from build123d import *

# Parameters (mm, degrees)
F1_DEPTH = 7


with BuildPart() as f1:
    # F0 (on Top) → F1 (new body)
    with BuildSketch(Plane.XY):
        with BuildLine():
            Line((41.277483, 14.2875), (0, 14.2875))
            ThreePointArc((0, 14.2875), (-7.9375, 6.35), (0, -1.5875))
            Line((0, -1.5875), (41.277483, -1.5875))
            ThreePointArc((41.277483, -1.5875), (49.214983, 6.35), (41.277483, 14.2875))
        make_face()
        with BuildLine():
            Line((41.277483, 0), (0, 0))
            ThreePointArc((0, 0), (-6.35, 6.35), (0, 12.7))
            Line((0, 12.7), (41.277483, 12.7))
            ThreePointArc((41.277483, 12.7), (47.627483, 6.35), (41.277483, 0))
        make_face(mode=Mode.SUBTRACT)
    extrude(amount=F1_DEPTH)


solid = f1.part
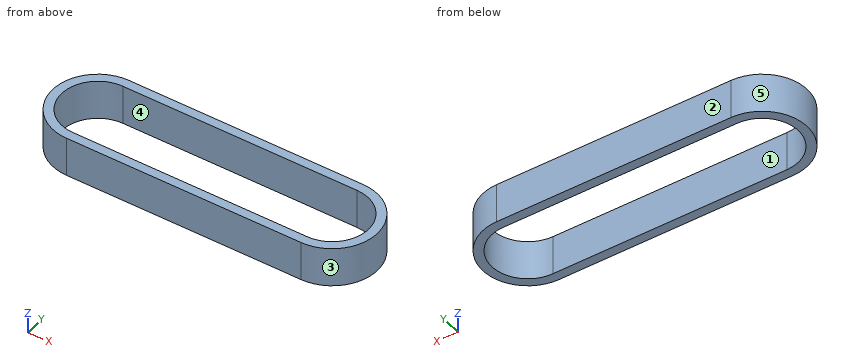
Could you check a few things on this model? Use its own coordinates, in mm. Face numbers are marked on the shaded views. A direction names the side the tool comes from. Round coordinates to 2 decimals unless told otherwise and drop trailing zeros. Loops run counter-clockwise (first coordinate to the right, second up) from the corner with the lowest first, then second, coordinate; pieces in that order, holes last. Notation, with made-up numbers: (-10, 1) - (2, 1) arc R15 ccw to (2, 30) - close; hole circle Ø9 at (-12, 9). An arc over 180 degrees is marked (long way). Write item = value, one per line.
1) Imagine slicing it at A-A (y = 6.35). Please give me the cut outline in (x, z), and give its area (3 significant figures).
Computed:
outline = (-7.94, 0) - (-6.35, 0) - (-6.35, 7) - (-7.94, 7) - close; (47.63, 0) - (49.21, 0) - (49.21, 7) - (47.63, 7) - close
area = 22.2 mm2
2) I'm going to push flat-ended pins straight in: P1, Ø1, axis at y = 3.5, z = 4.5, coming from the -X side; P2, Ø3, axis at y = 4.5, z = 1.5, coming from the -X side. Where does each tip first touch, or does it pass through?
Computed:
P1 = -7.58
P2 = -7.93
3) I need wall thicknesses on line 1 along Y through (x, z) = (6.5, 2.5); line 2 along X through (y, z) = (5.25, 1.75); line 3 along Y through (x, z) = (46, 1). Which ranges of each line are inside material? Lowest first, please. Write a range as from..to.
Computed:
line_1 = -1.59..0, 12.7..14.29
line_2 = -7.86..-6.25, 47.53..49.14
line_3 = -0.03..2.1, 10.6..12.73
4) Imagine slicing it at B-B (x = 40.5). Please give me the cut outline in (y, z).
Computed:
outline = (-1.59, 0) - (0, 0) - (0, 7) - (-1.59, 7) - close; (12.7, 0) - (14.29, 0) - (14.29, 7) - (12.7, 7) - close
5) On a 3-axis mill with a long thin cutter (end or side, diameter ignored), from which of +Z, -Z, +X, -X, +Y, -Y can I reach the whole of each face in a straight line? I mean the marked faces 4 and 5. Say none if no direction works.
Computed:
face_4 = +Z, -Z
face_5 = +Z, -Z, -X
6) If we mould it in two halves opening along Y, with no side actions, what happens to the marked faces 1, 2 and 3? For each: pulls with the +Y half, pulls with the -Y half, needs draft (parallel to the pull), parting line crosses it, or undercut.
Computed:
face_1 = undercut
face_2 = pulls with the +Y half
face_3 = parting line crosses it
